Build history of the part. All positions in model axes, mm. A direction names the side the tool comes from. Coordinates: 2 decimals unless noted, no trailing zeros. Loops run counter-clockwise (first coordinate to the right, second up) from the corner with the lowest first, then second, coordinate; pieces in that order, holes last.
(1) Wall check: L1, parallel to Z at x = 44, y = -1.9; L2, parallel to Z at x = 22, y = -0.25; L3, parallel to X at y = -1.65, z = 85.5. Give the ranges that are in metal, low to high.
(2) Tool access for faces 4 (the face through (1.83, -2.28, 56.44)), 5 (the face through (52.07, -1.61, 76.04)): list every direction of +Z, -Z, +X, -X, +Y, -Y with a clear straight run to the whole face (end or side of a thin tool).
(3) Slice it at D-D (z = 10.5). Give the cut face in (x, y) (3 decimals), and give its area (3 significant figures).
(4) Slice it at A-A (x = 41). Give the cut face in (y, z) (3 decimals).
(5) Slice it at C-C (y = -2). Give the number of separate pieces and of enclosed holes in the cut face, and give its area (3 significant figures).
(6) Slice it at B-B (z = 39). Give the cut face in (x, y) (3 decimals), and give its area (3 significant figures).
(7) Two-plate mould, pull along Z, no slides. Class faces 1 (the face through (35, -3.175, 58)), 2 (the face through (24.915, -1.61, 88.291)), 3 (the face through (34.52, -2.28, 112.47)): pulls with the +Z half, pulls with the -Z half, needs draft (parallel to the pull), parting line crosses it, or undercut.
(8) Flat gauge pin, fed straight in: P1, Ø1.6, axis at x = 38.5, y = -1, coming from the -Z side. Where does the tip first touch, or does it go through?
from build123d import *

# Parameters (mm, degrees)
F1_DEPTH     = 3.175
F2_T1_DEPTH  = 57.15
F2_T3_DEPTH  = 101.6
F2_T6_ANGLE  = 90
F2_T8_ANGLE  = 90
F2_T10_ANGLE = 90
F2_T12_ANGLE = 90
F4_DEPTH     = 25.4


# Not quite as in the source:
# - a fillet or chamfer that OpenCascade refuses, or shapes differently, is made with other operations: its cross-section is extruded or revolved along the edge and cut away or added


with BuildPart() as f1:
    # F0 (on Front) → F1 (new body)
    with BuildSketch(Plane.XZ):
        with BuildLine():
            ThreePointArc((0, 6.35), (1.8598719395, 1.8598719395), (6.35, 0))
            Line((6.35, 0), (63.5, 0))
            ThreePointArc((63.5, 0), (67.9901280605, 1.8598719395), (69.85, 6.35))
            Line((69.85, 6.35), (69.85, 107.95))
            ThreePointArc((69.85, 107.95), (67.9901280605, 112.4401280605), (63.5, 114.3))
            Line((63.5, 114.3), (6.35, 114.3))
            ThreePointArc((6.35, 114.3), (1.8598719395, 112.4401280605), (0, 107.95))
            Line((0, 107.95), (0, 6.35))
        make_face()
    extrude(amount=F1_DEPTH)

    # F2: fillet of radius 5.08 on 1 edges, made by hand

    # F2_s2 → F2_t1 (cut)
    with BuildSketch(Plane.YZ.offset(6.35)):
        with BuildLine():
            ThreePointArc((0, 114.3), (-2.3071134838, 112.4305202921), (-3.175, 109.5907139607))
            Line((-3.175, 109.5907139607), (-3.175, 114.3))
            Line((-3.175, 114.3), (0, 114.3))
        make_face()
        with BuildLine():
            ThreePointArc((0, 0), (-2.3071134838, 1.8694797079), (-3.175, 4.7092860393))
            Line((-3.175, 4.7092860393), (-3.175, 0))
            Line((-3.175, 0), (0, 0))
        make_face()
    extrude(amount=F2_T1_DEPTH, mode=Mode.SUBTRACT)

    # F2_s4 → F2_t3 (cut)
    with BuildSketch(Plane.XY.offset(6.35)):
        with BuildLine():
            ThreePointArc((0, 0), (1.8694797079, -2.3071134838), (4.7092860393, -3.175))
            Line((4.7092860393, -3.175), (0, -3.175))
            Line((0, -3.175), (0, 0))
        make_face()
        with BuildLine():
            ThreePointArc((69.85, 0), (67.9805202921, -2.3071134838), (65.1407139607, -3.175))
            Line((65.1407139607, -3.175), (69.85, -3.175))
            Line((69.85, -3.175), (69.85, 0))
        make_face()
    extrude(amount=F2_T3_DEPTH, mode=Mode.SUBTRACT)

    # F2_s5 → F2_t6 (revolve, cut)
    with BuildSketch(Plane.XY.offset(107.95)):
        with BuildLine():
            ThreePointArc((69.85, 0), (67.9805202921, -2.3071134838), (65.1407139607, -3.175))
            Line((65.1407139607, -3.175), (69.85, -3.175))
            Line((69.85, -3.175), (69.85, 0))
        make_face()
    revolve(axis=Axis((63.5, -3.175, 107.95), (0, -1, 0)), revolution_arc=F2_T6_ANGLE, mode=Mode.SUBTRACT)

    # F2_s7 → F2_t8 (revolve, cut)
    with BuildSketch(Plane.YZ.offset(6.35)):
        with BuildLine():
            ThreePointArc((0, 114.3), (-2.3071134838, 112.4305202921), (-3.175, 109.5907139607))
            Line((-3.175, 109.5907139607), (-3.175, 114.3))
            Line((-3.175, 114.3), (0, 114.3))
        make_face()
    revolve(axis=Axis((6.35, -3.175, 107.95), (0, -1, 0)), revolution_arc=F2_T8_ANGLE, mode=Mode.SUBTRACT)

    # F2_s9 → F2_t10 (revolve, cut)
    with BuildSketch(Plane.XY.offset(6.35)):
        with BuildLine():
            ThreePointArc((0, 0), (1.8694797079, -2.3071134838), (4.7092860393, -3.175))
            Line((4.7092860393, -3.175), (0, -3.175))
            Line((0, -3.175), (0, 0))
        make_face()
    revolve(axis=Axis((6.35, -3.175, 6.35), (0, -1, 0)), revolution_arc=F2_T10_ANGLE, mode=Mode.SUBTRACT)

    # F2_s11 → F2_t12 (revolve, cut)
    with BuildSketch(Plane.YZ.offset(63.5)):
        with BuildLine():
            ThreePointArc((0, 0), (-2.3071134838, 1.8694797079), (-3.175, 4.7092860393))
            Line((-3.175, 4.7092860393), (-3.175, 0))
            Line((-3.175, 0), (0, 0))
        make_face()
    revolve(axis=Axis((63.5, -3.175, 6.35), (0, -1, 0)), revolution_arc=F2_T12_ANGLE, mode=Mode.SUBTRACT)

    # F3 (on face) → F4 (cut)
    with BuildSketch(Plane.XZ.offset(3.175)):
        with BuildLine():
            ThreePointArc((27.628852542, 88.9), (24.879221885, 88.2738126498), (22.6718853808, 86.51875))
            ThreePointArc((22.6718853808, 86.51875), (19.05, 76.2), (22.6718853808, 65.88125))
            ThreePointArc((22.6718853808, 65.88125), (24.879221885, 64.1261873502), (27.628852542, 63.5))
            Line((27.628852542, 63.5), (43.491147458, 63.5))
            ThreePointArc((43.491147458, 63.5), (46.240778115, 64.1261873502), (48.4481146192, 65.88125))
            ThreePointArc((48.4481146192, 65.88125), (52.07, 76.2), (48.4481146192, 86.51875))
            ThreePointArc((48.4481146192, 86.51875), (46.240778115, 88.2738126498), (43.491147458, 88.9))
            Line((43.491147458, 88.9), (27.628852542, 88.9))
        make_face()
        with BuildLine():
            ThreePointArc((22.6718853808, 27.78125), (24.879221885, 26.0261873502), (27.628852542, 25.4))
            Line((27.628852542, 25.4), (43.491147458, 25.4))
            ThreePointArc((43.491147458, 25.4), (46.240778115, 26.0261873502), (48.4481146192, 27.78125))
            ThreePointArc((48.4481146192, 27.78125), (52.07, 38.1), (48.4481146192, 48.41875))
            ThreePointArc((48.4481146192, 48.41875), (46.240778115, 50.1738126498), (43.491147458, 50.8))
            Line((43.491147458, 50.8), (27.628852542, 50.8))
            ThreePointArc((27.628852542, 50.8), (24.879221885, 50.1738126498), (22.6718853808, 48.41875))
            ThreePointArc((22.6718853808, 48.41875), (19.05, 38.1), (22.6718853808, 27.78125))
        make_face()
    extrude(amount=-F4_DEPTH, mode=Mode.SUBTRACT)


solid = f1.part
Response values:
1. L1: z = 1.34 to 25.42, 50.78 to 63.52, 88.88 to 112.96
1. L2: z = 0.11 to 28.68, 47.52 to 66.78, 85.62 to 114.19
1. L3: x = 1.08 to 21.92, 49.2 to 68.77
2. face 4: +Z, -Z, -X, -Y
2. face 5: +Y, -Y
3. outline: (0, 0) arc R5.08 ccw to (4.709, -3.175) - (65.141, -3.175) arc R5.08 ccw to (69.85, 0) - close
3. area: 214 mm2
4. outline: (-3.175, 4.709) arc R5.08 ccw to (0, 0) - (0, 25.4) - (-3.175, 25.4) - close; (-3.175, 50.8) - (0, 50.8) - (0, 63.5) - (-3.175, 63.5) - close; (-3.175, 88.9) - (0, 88.9) - (0, 114.3) arc R5.08 ccw to (-3.175, 109.591) - close
5. separate pieces: 1
5. enclosed holes: 2
5. area: 5,950 mm2
6. outline: (0, 0) arc R5.08 ccw to (4.709, -3.175) - (19.075, -3.175) - (19.075, 0) - close; (52.045, -3.175) - (65.141, -3.175) arc R5.08 ccw to (69.85, 0) - (52.045, 0) - close
6. area: 109 mm2
7. face 1: needs draft
7. face 2: undercut
7. face 3: pulls with the +Z half
8. P1: stops at z = 0.09
